Model file for the job. Use its own axes, mm. A direction names the side the tool comes from. Coordinates: 2 decimals unless noted, no trailing zeros. Order: outer loops, then holes, each group sorted by start corner. A loop starts at its lowest first (then second) coordinate and runs counter-clockwise, first axis right, second up. Notation, with made-up numbers: M 34,-10.75 L 56,-10.75 A8 cw 56,0.25 Z; hole C -8.75,-7 d5. An arc over 180 degrees is marked long. Return JSON: item names as keys, results as strings.
```python
from build123d import *

# Parameters (mm, degrees)
F0_R      = 60
F1_DEPTH  = 10
F2_W      = 20
F2_H      = 10
F3_DEPTH  = 10
F5_D      = 2.5
F7_D      = 2.5
F9_D      = 2.5
F11_DEPTH = 10.001
F13_DEPTH = 25


with BuildPart() as f1:
    # F0 (on Front) → F1 (new body)
    with BuildSketch(Plane.XZ):
        Circle(F0_R)
    extrude(amount=F1_DEPTH)

    # F2 (on face) → F3 (join)
    with BuildSketch(Plane.XZ.offset(10)):
        with Locations((0, 63)):
            Rectangle(F2_W, F2_H)
        Polygon((-53.8897274573, -42.6602540378), (-45.2294734195, -37.6602540378), (-55.2294734195, -20.3397459622), (-63.8897274573, -25.3397459622), align=None)
        Polygon((63.8897274573, -25.3397459622), (55.2294734195, -20.3397459622), (45.2294734195, -37.6602540378), (53.8897274573, -42.6602540378), align=None)
    extrude(amount=-F3_DEPTH)

    # F5 (through all)
    with Locations(Plane(origin=(-10, 0, 0), x_dir=(0, -1, 0), z_dir=(-1, 0, 0))):
        with Locations((5, 63.5803989155)):
            Hole(F5_D / 2)

    # F7 (through all)
    with Locations(Plane(origin=(-5, 0, 8.6602540378), x_dir=(0.8660254038, 0, 0.5), z_dir=(-0.5, 0, 0.8660254038))):
        with Locations((-63.5803989155, -5)):
            Hole(F7_D / 2)

    # F9 (through all)
    with Locations(Plane(origin=(-5, 0, -8.6602540378), x_dir=(0.8660254038, 0, -0.5), z_dir=(-0.5, 0, -0.8660254038))):
        with Locations((63.5803989155, 5)):
            Hole(F9_D / 2)

    # F10 (on face) → F11 (cut, through all)
    with BuildSketch(Plane.XZ):
        Polygon((46.057395637, -38.3253619075), (-46.2041050196, -38.3253619075), (-47.8550866246, -60.4935437441), (42.8329333663, -62.1057748795), align=None)
    extrude(amount=F11_DEPTH, mode=Mode.SUBTRACT)

    # F12 (on face) → F13 (cut)
    with BuildSketch(Plane(origin=(0, 0, 0), x_dir=(-1, 0, 0), z_dir=(0, 1, 0))):
        Polygon((10, 59.160797831), (56.2347538298, -20.9201448777), (84.3601897359, -9.6184732392), (39.3041819334, 80.4935470223), align=None)
        Polygon((-56.2347538298, -20.9201448777), (-10, 59.160797831), (-43.3372279011, 71.7235354264), (-86.677499705, -3.3440173517), align=None)
    extrude(amount=-F13_DEPTH, mode=Mode.SUBTRACT)


solid = f1.part
```
Item 1: Saw through at C-C (z = 46.5). Write the cut outline in (x, y).
Check result:
{"outline": "M -17.31,-10 L 17.31,-10 L 17.31,0 L -17.31,0 Z"}
Item 2: Pull direction X, two halves, no side cores. Call faces 4 (the flat face through (33.44, -4.93, 18.56)), 5 (the cylindrical face through (-55.49, -6.11, -32.2)), 6 (the flat face through (-50.966, -6.181, -40.972)), 7 (the flat face through (-58.96, -5.07, -33.88)): +X half, -X half, draft (parallel to the pull), parting line (faces both ways), or undercut.
Check result:
{"face 4": "+X half", "face 5": "undercut", "face 6": "undercut", "face 7": "-X half"}
Item 3: Saw through at D-D (z = -33). Count the separate pieces of the cut face and the enclosed holes in it, and give its area (3 significant figures).
Check result:
{"separate pieces": "1", "enclosed holes": "2", "area": "1,180 mm2"}
Item 4: Saw through at B-B (x = -44.5). Write the cut outline in (y, z).
Check result:
{"outline": "M -10,-38.33 L 0,-38.33 L 0,-0.59 L -10,-0.59 Z"}
Item 5: Saw through at A-A (y = -8). Write the cut outline in (x, z), and give its area (3 significant figures).
Check result:
{"outline": "M -63.89,-25.34 L -53.89,-42.66 L -46.23,-38.24 A60 ccw -46.16,-38.33 L 46.06,-38.33 L 46.04,-38.48 A60 ccw 46.23,-38.24 L 53.89,-42.66 L 63.89,-25.34 L 56.23,-20.92 L 10,59.16 L 10,68 L -10,68 L -10,59.16 L -56.23,-20.92 Z", "area": "7,620 mm2"}
Item 6: 3-axis set-ups, long thin cutter, end or side, ignore diameter. For faces 1 (the flat face through (-10, -6, 65)), 2 (the flat face through (10, -6, 65)), 3 (the flat face through (1, -5, -38.325)): which of +Z, -Z, +X, -X, +Y, -Y reach the whole face in a straight line?
Check result:
{"face 1": "+Z, -X, +Y, -Y", "face 2": "+Z, +X, +Y, -Y", "face 3": "-Z, +Y, -Y"}
Item 7: Drop flat-ended pins along their axis: pin 1 Ø1 at (y, z) = (-4.5, -7) entering from +X; pin 2 Ø4 at (x, y) = (51, -2) entering from +Z; pin 3 Ø1 at (x, y) = (-16, -5.5) entering from -Z. Give the stop position or say it passes through.
Check result:
{"pin 1": "stops at x = 48.49", "pin 2": "stops at z = -8.39", "pin 3": "stops at z = -38.33"}
Item 8: Wall check: line 1 (Z direction, x = -3, y = -5); line 2 (X direction, y = -7.75, z = 60.5); line 3 (Z direction, x = 1, y = -1.5). Give the ranges that are in metal, low to high.
Check result:
{"line 1": "z = -38.33 to 62.33, 64.83 to 68", "line 2": "x = -10 to 10", "line 3": "z = -38.33 to 68"}
